For this review, take the finished solid that the model builds, in its own axes (mm). Face numbers are marked on the shaded views. A direction names the side the tool comes from. Coordinates: 2 decimals unless noted, no trailing zeros. Loops run counter-clockwise (first coordinate to the right, second up) from the corner with the lowest first, then second, coordinate; pieces in that order, holes last. Notation, with made-up numbers: (33, 21.5) -> (85, 21.5) arc R8 cw to (85, 35.5) -> close; hole circle Ø6 at (83.25, 55.5). An arc over 180 degrees is marked (long way). Use a Markdown table: item, result.
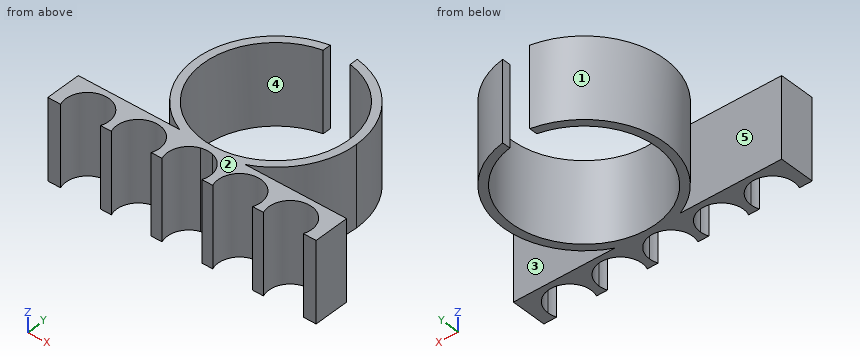
from build123d import *

# Parameters (mm, degrees)
F0_R     = 17.145
F1_DEPTH = 19.05
F2_DEPTH = 25.4
F3_W     = 6.35
F3_H     = 30.0934736039
F4_DEPTH = 25.4


# Not quite as in the source:
# - a feature names something its author has since deleted; it is built from what else it names


with BuildPart() as f1:
    # F0 (on Top) → F1 (new body)
    with BuildSketch(Plane.XY):
        with BuildLine():
            ThreePointArc((7.7574028515, -17.399), (15.9793777151, -10.3712095649), (19.05, 0))
            ThreePointArc((19.05, 0), (-10.3712095649, 15.9793777151), (-7.7574028515, -17.399))
            Line((-7.7574028515, -17.399), (7.7574028515, -17.399))
        make_face()
        Circle(F0_R, mode=Mode.SUBTRACT)
        with BuildLine():
            Line((7.7574028515, -17.399), (-7.7574028515, -17.399))
            ThreePointArc((-7.7574028515, -17.399), (-4.6557505543, -18.472316768), (-1.4158987787, -18.9973085106))
            ThreePointArc((-1.4158987787, -18.9973085106), (0, -18.796), (1.4158987787, -18.9973085106))
            ThreePointArc((1.4158987787, -18.9973085106), (4.6557505543, -18.472316768), (7.7574028515, -17.399))
        make_face()
        with BuildLine():
            Line((31.75, -17.399), (7.7574028515, -17.399))
            ThreePointArc((7.7574028515, -17.399), (4.6557505543, -18.472316768), (1.4158987787, -18.9973085106))
            ThreePointArc((1.4158987787, -18.9973085106), (4.0619678603, -20.8252923605), (5.08, -23.876))
            ThreePointArc((5.08, -23.876), (4.9864603217, -24.8463676933), (4.7092860393, -25.781))
            Line((4.7092860393, -25.781), (7.2907139607, -25.781))
            ThreePointArc((7.2907139607, -25.781), (11.0296323067, -18.8895396783), (17.08, -23.876))
            ThreePointArc((17.08, -23.876), (16.9864603217, -24.8463676933), (16.7092860393, -25.781))
            Line((16.7092860393, -25.781), (19.2907139607, -25.781))
            ThreePointArc((19.2907139607, -25.781), (23.0296323067, -18.8895396783), (29.08, -23.876))
            ThreePointArc((29.08, -23.876), (28.9864603217, -24.8463676933), (28.7092860393, -25.781))
            Line((28.7092860393, -25.781), (31.75, -25.781))
            Line((31.75, -25.781), (31.75, -17.399))
        make_face()
        with BuildLine():
            ThreePointArc((-1.4158987787, -18.9973085106), (-4.6557505543, -18.472316768), (-7.7574028515, -17.399))
            Line((-7.7574028515, -17.399), (-31.75, -17.399))
            Line((-31.75, -17.399), (-31.75, -25.781))
            Line((-31.75, -25.781), (-28.7092860393, -25.781))
            ThreePointArc((-28.7092860393, -25.781), (-24.9703676933, -18.8895396783), (-18.92, -23.876))
            ThreePointArc((-18.92, -23.876), (-19.0135396783, -24.8463676933), (-19.2907139607, -25.781))
            Line((-19.2907139607, -25.781), (-16.7092860393, -25.781))
            ThreePointArc((-16.7092860393, -25.781), (-12.9703676933, -18.8895396783), (-6.92, -23.876))
            ThreePointArc((-6.92, -23.876), (-7.0135396783, -24.8463676933), (-7.2907139607, -25.781))
            Line((-7.2907139607, -25.781), (-4.7092860393, -25.781))
            ThreePointArc((-4.7092860393, -25.781), (-4.5699113579, -21.6573720049), (-1.4158987787, -18.9973085106))
        make_face()
    extrude(amount=F1_DEPTH)

    # F0 (on Top) → F2 (cut)
    with BuildSketch(Plane.XY):
        with BuildLine():
            Line((-16.7092860393, -25.781), (-7.2907139607, -25.781))
            ThreePointArc((-7.2907139607, -25.781), (-7.0135396783, -24.8463676933), (-6.92, -23.876))
            ThreePointArc((-6.92, -23.876), (-12.9703676933, -18.8895396783), (-16.7092860393, -25.781))
        make_face()
        with BuildLine():
            ThreePointArc((-18.92, -23.876), (-24.9703676933, -18.8895396783), (-28.7092860393, -25.781))
            Line((-28.7092860393, -25.781), (-19.2907139607, -25.781))
            ThreePointArc((-19.2907139607, -25.781), (-19.0135396783, -24.8463676933), (-18.92, -23.876))
        make_face()
        with BuildLine():
            ThreePointArc((17.08, -23.876), (11.0296323067, -18.8895396783), (7.2907139607, -25.781))
            Line((7.2907139607, -25.781), (16.7092860393, -25.781))
            ThreePointArc((16.7092860393, -25.781), (16.9864603217, -24.8463676933), (17.08, -23.876))
        make_face()
    extrude(amount=F2_DEPTH, mode=Mode.SUBTRACT)

    # F3 (on Top) → F4 (cut)
    with BuildSketch(Plane.XY):
        with Locations((-0.1380435133, 15.0467368019)):
            Rectangle(F3_W, F3_H)
    extrude(amount=F4_DEPTH, mode=Mode.SUBTRACT)


solid = f1.part
(1) Take a section at A-A on y = -7. Write out the cut boundary in (x, z).
Found:
| item | result |
|---|---|
| outline | (-17.72, 0) -> (-15.65, 0) -> (-15.65, 19.05) -> (-17.72, 19.05) -> close; (15.65, 0) -> (17.72, 0) -> (17.72, 19.05) -> (15.65, 19.05) -> close |
(2) Mouldability with a two-part tool opening along Y and no side actions: class the marked faces 1 and 2 as pulls with the +Y half, pulls with the -Y half, needs draft (parallel to the pull), parting line crosses it, or undercut.
Found:
| item | result |
|---|---|
| face 1 | undercut |
| face 2 | needs draft |
(3) For pin 1 Ø0.6 at (y, z) = (17.5, 8) entering from +X; pin 2 Ø8 at (x, z) = (-19, 2.5) entering from +Y; pin 3 Ø1.5 at (x, z) = (0.5, 5) entering from +Y, all flat-tipped, find the tip position at first contact; note any pin that passes through.
Found:
| item | result |
|---|---|
| pin 1 | stops at x = 8.19 |
| pin 2 | stops at y = 11.74 |
| pin 3 | stops at y = -17.1 |
(4) Take a section at D-D on y = -21. Write out the cut boundary in (x, z), plus the area to 3 significant figures.
Found:
| item | result |
|---|---|
| outline | (-31.75, 0) -> (-28.19, 0) -> (-28.19, 19.05) -> (-31.75, 19.05) -> close; (-19.81, 0) -> (-16.19, 0) -> (-16.19, 19.05) -> (-19.81, 19.05) -> close; (-7.81, 0) -> (-4.19, 0) -> (-4.19, 19.05) -> (-7.81, 19.05) -> close; (4.19, 0) -> (7.81, 0) -> (7.81, 19.05) -> (4.19, 19.05) -> close; (16.19, 0) -> (19.81, 0) -> (19.81, 19.05) -> (16.19, 19.05) -> close; (28.19, 0) -> (31.75, 0) -> (31.75, 19.05) -> (28.19, 19.05) -> close |
| area | 412 mm^2 |
(5) For line 1 along Y through (x, z) = (-11.5, 9.5); line 2 along Y through (x, z) = (12, 10.75); line 3 along X through (y, z) = (-0.5, 11), list the stretches that pass through material, from the lowest coordinate up.
Found:
| item | result |
|---|---|
| line 1 | y = -18.82 to -17.4, -15.19 to -12.72, 12.72 to 15.19 |
| line 2 | y = -18.8 to -17.4, -14.8 to -12.25, 12.25 to 14.8 |
| line 3 | x = -19.04 to -17.14, 17.14 to 19.04 |
(6) Take a section at C-C on z = 12. Write out the cut boundary in (x, y) (3 decimals).
Found:
| item | result |
|---|---|
| outline | (-31.75, -25.781) -> (-28.709, -25.781) arc R5.08 cw (long way) to (-19.291, -25.781) -> (-16.709, -25.781) arc R5.08 cw (long way) to (-7.291, -25.781) -> (-4.709, -25.781) arc R5.08 cw (long way) to (4.709, -25.781) -> (7.291, -25.781) arc R5.08 cw (long way) to (16.709, -25.781) -> (19.291, -25.781) arc R5.08 cw (long way) to (28.709, -25.781) -> (31.75, -25.781) -> (31.75, -17.399) -> (7.757, -17.399) arc R19.05 ccw to (3.037, 18.806) -> (3.037, 16.874) arc R17.145 cw (long way) to (-3.313, 16.822) -> (-3.313, 18.76) arc R19.05 ccw to (-7.757, -17.399) -> (-31.75, -17.399) -> close |
(7) For the marked faces 3, 4 and 5, list the 3-axis set-ups (+Z, -Z, +X, -X, +Y, -Y) from which the entire face can be reached by the end or side of a thin tool; tool diameter is ignored.
Found:
| item | result |
|---|---|
| face 3 | +Z, -Z, +X |
| face 4 | +Z, -Z |
| face 5 | +Z, -Z, -X |
(8) Take a section at B-B on x = -12. Write out the cut boundary in (y, z), plus the area to 3 significant figures.
Found:
| item | result |
|---|---|
| outline | (-18.8, 0) -> (-17.4, 0) -> (-17.4, 19.05) -> (-18.8, 19.05) -> close; (-14.8, 0) -> (-12.25, 0) -> (-12.25, 19.05) -> (-14.8, 19.05) -> close; (12.25, 0) -> (14.8, 0) -> (14.8, 19.05) -> (12.25, 19.05) -> close |
| area | 124 mm^2 |
